Solid Edge part; units mm, degrees
sketch "Sketch1" plane through (0, 0, 0) normal (0, 0, 1) x (1, 0, 0)
  line L0 (-12.5, -12.5) -> (12.5, -12.5)
  line L1 (12.5, -12.5) -> (12.5, 12.5)
  line L2 (12.5, 12.5) -> (-12.5, 12.5)
  line L3 (-12.5, 12.5) -> (-12.5, -12.5)
  dimension "D1" = 12.5
  dimension "D2" = 12.5
extrude "Protrusion1" add sketch "Sketch1" along normal mid plane 4
fillet "Verrundung_1" radius 12.5 2 edges at (12.5, 12.5, 0) (-12.5, 12.5, 0)
sketch "Sketch2" plane through (0, 0, 2) normal (0, 0, 1) x (1, 0, 0)
  circle A0 centre (0, 0) radius 9
extrude "Extrusionsausschnitt_1" cut sketch "Sketch2" against normal blind 16
sketch "Sketch3" plane through (0, 0, 2) normal (0, 0, 1) x (1, 0, 0)
  line L0 (-2.505, -12.5) -> (2.505, -12.5)
  line L1 (2.505, -12.5) -> (2.505, -16.5)
  line L2 (2.505, -16.5) -> (-2.505, -16.5)
  line L3 (-2.505, -16.5) -> (-2.505, -12.5)
  line L4 (7.49, -12.5) -> (12.5, -12.5)
  line L5 (12.5, -12.5) -> (12.5, -16.5)
  line L6 (12.5, -16.5) -> (7.49, -16.5)
  line L7 (7.49, -16.5) -> (7.49, -12.5)
  line L8 (-12.5, -12.5) -> (-7.49, -12.5)
  line L9 (-7.49, -12.5) -> (-7.49, -16.5)
  line L10 (-7.49, -16.5) -> (-12.5, -16.5)
  line L11 (-12.5, -16.5) -> (-12.5, -12.5)
  dimension "D1" = 12.5
  dimension "D2" = 2.505
  dimension "D3" = 7.49
  dimension "D4" = 12.5
  dimension "D5" = 2.505
  dimension "D6" = 7.49
extrude "Extrusionsausprägung_2" add sketch "Sketch3" against normal blind 4
properties material "Holz, Kiefer"
Geometry check sheet. Reference: the model listing, model coordinates, mm. A direction names the side the tool comes from. Give positions to 0.01 mm unless a question says otherwise; leave off trailing zeros. Order: outer loops, then holes, each group sorted by start corner. A loop starts at its lowest first (then second) coordinate and runs counter-clockwise, first axis right, second up. Notation, with made-up numbers: (34.25, 14) - (39.25, 14) arc R3 cw to (39.25, 18) - close; hole circle Ø3 at (-28.75, 82). An arc over 180 degrees is marked (long way). Answer as a JSON object with one key per item and string values.
(1) Cross-section at C-C (x = 7). Record the cut outline in (y, z), then the cut area to 3 significant figures.
Report:
{"outline": "(-12.5, -2) - (-5.66, -2) - (-5.66, 2) - (-12.5, 2) - close; (5.66, -2) - (10.36, -2) - (10.36, 2) - (5.66, 2) - close", "area": "46.2 mm^2"}
(2) Cross-section at B-B (y = 3.5). Record the cut outline in (x, z), then the cut area to 3 significant figures.
Report:
{"outline": "(-12, -2) - (-8.29, -2) - (-8.29, 2) - (-12, 2) - close; (8.29, -2) - (12, -2) - (12, 2) - (8.29, 2) - close", "area": "29.7 mm^2"}
(3) Cross-section at D-D (x = -9.5). Record the cut outline in (y, z), then the cut area to 3 significant figures.
Report:
{"outline": "(-16.5, -2) - (8.12, -2) - (8.12, 2) - (-16.5, 2) - close", "area": "98.5 mm^2"}
(4) Draft check along X on faces 1 (the flat face through (12.5, -8, 0)), 2 (the cylindrical face through (-8.94, 8.74, -0.03)), 3 (the flat face through (0, -16.5, 0)), 4 (the flat face through (-5, -12.5, 0)). Enter one of: released by +X, released by -X, zero draft, split by the parting line, or undercut.
Report:
{"face 1": "released by +X", "face 2": "released by -X", "face 3": "zero draft", "face 4": "undercut"}
(5) Depth check by flat-ended pin: pin 1 Ø6 at (x, y) = (-0.5, 4) entering from +Z; pin 2 Ø2 at (x, z) = (-4, 0) entering from -Y; pin 3 Ø2 at (y, z) = (8, -0.5) entering from +X; pin 4 Ø2 at (y, z) = (3.5, 0) entering from -X. Enter the tip coordinate at first touch or a pass-through.
Report:
{"pin 1": "through", "pin 2": "y = -12.5", "pin 3": "x = 10.36", "pin 4": "x = -12.25"}
(6) Tool access check on faces 5 (the flat face through (5, -12.5, 0)), 6 (the flat face through (-6, -8, 2)). Record the directions out of +Z, -Z, +X, -X, +Y, -Y that give a thin tool (end or side, any length) a straight path to the whole face; none if there is none.
Report:
{"face 5": "+Z, -Z, -Y", "face 6": "+Z, +X, -X, +Y, -Y"}
(7) Material ranges on line 1 (X direction, y = -14.5, z = 1.85) (3 decimals); line 2 (Y direction, x = 0, z = 0.6); line 3 (X direction, y = 0.25, z = 0), recorded low to high.
Report:
{"line 1": "-12.5 to -7.49, -2.505 to 2.505, 7.49 to 12.5", "line 2": "-16.5 to -9, 9 to 12.5", "line 3": "-12.5 to -9, 9 to 12.5"}
